from build123d import *

# Parameters (mm, degrees)
F0_R     = 11.049
F1_DEPTH = 6.985
F2_SIZE  = 1.27


with BuildPart() as f1:
    # F0 (on Top) → F1 (new body)
    with BuildSketch(Plane.XY):
        with BuildLine():
            ThreePointArc((4.999437, 13.992695), (1.765902, 16.583511), (0.818767, 20.617245))
            ThreePointArc((0.818767, 20.617245), (-19.4945, 33.765464), (-18.264442, 9.599549))
            ThreePointArc((-18.264442, 9.599549), (-15.244693, 6.762439), (-14.617748, 2.666708))
            ThreePointArc((-14.617748, 2.666708), (-14.859, 0), (-14.617748, -2.666708))
            ThreePointArc((-14.617748, -2.666708), (-15.244693, -6.762439), (-18.264442, -9.599549))
            ThreePointArc((-18.264442, -9.599549), (-19.4945, -33.765464), (0.818767, -20.617245))
            ThreePointArc((0.818767, -20.617245), (1.765902, -16.583511), (4.999437, -13.992695))
            ThreePointArc((4.999437, -13.992695), (7.4295, -12.868271), (9.618311, -11.325987))
            ThreePointArc((9.618311, -11.325987), (13.478791, -9.821072), (17.445675, -11.017696))
            ThreePointArc((17.445675, -11.017696), (38.989, 0), (17.445675, 11.017696))
            ThreePointArc((17.445675, 11.017696), (13.478791, 9.821072), (9.618311, 11.325987))
            ThreePointArc((9.618311, 11.325987), (7.4295, 12.868271), (4.999437, 13.992695))
        make_face()
        with Locations((-12.7, -21.997045)):
            Circle(F0_R, mode=Mode.SUBTRACT)
        Circle(F0_R, mode=Mode.SUBTRACT)
        with Locations((25.4, 0)):
            Circle(F0_R, mode=Mode.SUBTRACT)
        with Locations((-12.7, 21.997045)):
            Circle(F0_R, mode=Mode.SUBTRACT)
    extrude(amount=F1_DEPTH)

    # F2
    f2_edges = [f1.edges().sort_by_distance(p)[0] for p in [
        (-19.4945, -33.765464, 6.985),
        (1.765902, -16.583511, 0),
    ]]
    chamfer(f2_edges, length=F2_SIZE)


solid = f1.part
The model under review builds one solid part; all positions refer to its coordinate system, in mm. A direction names the side the tool comes from. Round coordinates to 2 decimals unless told otherwise and drop trailing zeros. Loops run counter-clockwise (first coordinate to the right, second up) from the corner with the lowest first, then second, coordinate; pieces in that order, holes last. Notation, with made-up numbers: M 16,-18 L 65,-18 A23 cw 65,18 Z; hole C -15.75,-11.75 d1. An arc over 180 degrees is marked long. Answer as CSV lines item,"result". Start each with the question number.
Item 1: Wall thickness on line 1 (Y direction, x = -12.7, z = 5); line 2 (Y direction, x = 25.4, z = 4.75); line 3 (X direction, y = -4, z = 2.25): over which ranges is each line inside the solid? List them lowest first. Write a range as [from, to].
Item 2: Consider section B-B (z = 4.5). Write out the cut boundary in (x, y), then the cut area to 3 significant figures.
Item 3: Mouldability with a two-part tool opening along X and no side actions: class faces 1 (the face through (-15.217, -6.71, 3.461)), 2 (the face through (-19.13, 33.97, 3.46)), 3 (the face through (7.46, 12.85, 3.46)), 4 (the face through (14.36, 0.49, 3.44)) as released by +X, released by -X, zero draft, split by the parting line, or undercut.
Item 4: Insertion check: P1, Ø2, axis at x = -15.5, z = 4, coming from the +Y side; P2, Ø1, axis at y = -15, z = 2.5, coming from the -X side; P3, Ø1.5, axis at y = 24.5, z = 2.5, coming from the -X side. Each pin has a flat end and moves straight along its axis. Give the tip position at first contact, or say it passes through.
Item 5: For faces 5 (the face through (1.735, -16.634, 3.461)), 6 (the face through (13.54, 9.82, 3.46)), 7 (the face through (7.397, -12.887, 3.461)), list the 3-axis set-ups (+Z, -Z, +X, -X, +Y, -Y) from which the entire face can be reached by the end or side of a thin tool; tool diameter is ignored.
Item 6: Consider section A-A (y = 0). Write out the cut boundary in (x, z) (3 decimals).
Item 7: Consider section C-C (x = -9.5). State how many separate pieces and enclosed holes the cut face has, then the cut area to 3 significant figures.
Answer:
1,line 1,"y = [-35.59, -33.05], [-10.95, 10.95], [33.05, 35.59]"
1,line 2,"y = [-13.59, -11.05], [11.05, 13.59]"
1,line 3,"x = [-14.52, -10.3], [10.3, 15.1], [35.7, 38.39]"
2,outline,"M -18.26,-9.6 A13.59 ccw long 0.82,-20.62 A6.35 cw 5,-13.99 A14.86 ccw 9.62,-11.33 A6.35 cw 17.45,-11.02 A13.59 ccw long 17.45,11.02 A6.35 cw 9.62,11.33 A14.86 ccw 5,13.99 A6.35 cw 0.82,20.62 A13.59 ccw long -18.26,9.6 A6.35 cw -14.62,2.67 A14.86 ccw -14.62,-2.67 A6.35 cw Z; hole C -12.7,-22 d22.1; hole C -12.7,22 d22.1; hole C 0,0 d22.1; hole C 25.4,0 d22.1"
2,area,"873 mm^2"
3,face 1,"released by -X"
3,face 2,"split by the parting line"
3,face 3,"undercut"
3,face 4,"undercut"
4,P1,"stops at y = 35.47"
4,P2,"stops at x = -24.64"
4,P3,"stops at x = -26.18"
5,face 5,"+Z, -Z, +X"
5,face 6,"+Z, -Z, +Y"
5,face 7,"+Z, -Z, -Y"
6,outline,"M -14.859,1.27 L -13.589,0 L -11.049,0 L -11.049,6.985 L -13.589,6.985 L -14.859,5.715 Z; M 11.049,0 L 14.351,0 L 14.351,6.985 L 11.049,6.985 Z; M 36.449,0 L 37.719,0 L 38.989,1.27 L 38.989,5.715 L 37.719,6.985 L 36.449,6.985 Z"
7,separate pieces,"4"
7,enclosed holes,"0"
7,area,"114 mm^2"
